Build history of the part. All positions in model axes, mm. A direction names the side the tool comes from. Round coordinates to 2 decimals unless told otherwise and drop trailing zeros. Write each loop counter-clockwise with the first axis right and the second up, starting at its lowest first coordinate (ties: lowest second). Pieces come first, ordered by that corner, then holes. Notation, with made-up numbers: M 26,60.25 L 65,60.25 A12 cw 65,69.25 Z; hole C 9,61.25 d4. An arc over 180 degrees is marked long. Write item = value, one per line.
from build123d import *

# Parameters (mm, degrees)
SKETCH_1_R      = 2.05
SKETCH_1_R_2    = 3
SKETCH_1_R_3    = 1.25
SKETCH_1_W      = 2.1
SKETCH_1_H      = 8.1
EXTRUDE_1_DEPTH = 2
FILLET_1_R      = 1.3
FILLET_2_R      = 2


with BuildPart() as part:
    # 草图1 → 凸台-拉伸1 (new body)
    with BuildSketch(Plane.XY):
        with BuildLine():
            Line((32.115707856, 28), (32.115707856, 22.85))
            Line((32.115707856, 22.85), (30.015707856, 22.85))
            Line((30.015707856, 22.85), (30.015707856, 28))
            Line((30.015707856, 28), (-29.075, 28))
            Line((-29.075, 28), (-38.998995168, 22.002009663))
            ThreePointArc((-38.998995168, 22.002009663), (-52.370174504, 17.472835843), (-60.236366221, 5.75))
            Line((-60.236366221, 5.75), (-79.631279411, 5.75))
            Line((-79.631279411, 5.75), (-79.631279411, -5.75))
            Line((-79.631279411, -5.75), (-60.236366221, -5.75))
            ThreePointArc((-60.236366221, -5.75), (-52.370174504, -17.472835843), (-38.998995168, -22.002009663))
            Line((-38.998995168, -22.002009663), (-29.075, -28))
            Line((-29.075, -28), (30.015707856, -28))
            Line((30.015707856, -28), (30.015707856, -22.85))
            Line((30.015707856, -22.85), (32.115707856, -22.85))
            Line((32.115707856, -22.85), (32.115707856, -28))
            Line((32.115707856, -28), (36.001004832, -28))
            Line((36.001004832, -28), (36.001004832, -26.017733681))
            Line((36.001004832, -26.017733681), (58.888331717, -26.017733681))
            Line((58.888331717, -26.017733681), (58.888331717, -21.401911511))
            Line((58.888331717, -21.401911511), (36.001004832, -21.401911511))
            Line((36.001004832, -21.401911511), (36.001004832, 28))
            Line((36.001004832, 28), (32.115707856, 28))
        make_face()
        with Locations((31.065707856, 15)):
            Circle(SKETCH_1_R, mode=Mode.SUBTRACT)
        with Locations(Location((31.065707856, -15, 0), (0, 0, 180))):
            Circle(SKETCH_1_R, mode=Mode.SUBTRACT)
        with Locations((-38.998995168, 0)):
            Circle(SKETCH_1_R_2, mode=Mode.SUBTRACT)
        with Locations((-38.998995168, -11.5)):
            Circle(SKETCH_1_R_3, mode=Mode.SUBTRACT)
        with Locations((-48.958287312, -5.75)):
            Circle(SKETCH_1_R_3, mode=Mode.SUBTRACT)
        with Locations((-48.958287312, 5.75)):
            Circle(SKETCH_1_R_3, mode=Mode.SUBTRACT)
        with Locations((-38.998995168, 11.5)):
            Circle(SKETCH_1_R_3, mode=Mode.SUBTRACT)
        with Locations((-29.039703025, 5.75)):
            Circle(SKETCH_1_R_3, mode=Mode.SUBTRACT)
        with Locations((-29.039703025, -5.75)):
            Circle(SKETCH_1_R_3, mode=Mode.SUBTRACT)
        with Locations((1.001004832, -25)):
            Circle(SKETCH_1_R, mode=Mode.SUBTRACT)
        with Locations((1.001004832, 25)):
            Circle(SKETCH_1_R, mode=Mode.SUBTRACT)
        with Locations((-74.958287312, 0)):
            Circle(SKETCH_1_R, mode=Mode.SUBTRACT)
        with Locations((31.065707856, 0)):
            Rectangle(SKETCH_1_W, SKETCH_1_H, mode=Mode.SUBTRACT)
        Polygon((2.100885183, -16.20323489), (23.065707856, -9.230000311), (23.065707856, 9.230000311), (2.100885183, 16.20323489), (-21.039703025, 1.3748119), (-21.039703025, -1.3748119), align=None, mode=Mode.SUBTRACT)
    extrude(amount=EXTRUDE_1_DEPTH)

    # 圆角1
    fillet_1_edges = [part.edges().sort_by_distance(p)[0] for p in [
        (-60.236366221, -5.75, 1),
        (-79.631279411, -5.75, 1),
        (-79.631279411, 5.75, 1),
        (-60.236366221, 5.75, 1),
        (30.015707856, 28, 1),
        (32.115707856, 28, 1),
        (32.115707856, -28, 1),
        (30.015707856, -28, 1),
    ]]
    fillet(fillet_1_edges, radius=FILLET_1_R)

    # 圆角2
    fillet_2_edges = [part.edges().sort_by_distance(p)[0] for p in [
        (-21.039703025, -1.3748119, 1),
        (2.100885183, -16.20323489, 1),
        (23.065707856, -9.230000311, 1),
        (23.065707856, 9.230000311, 1),
        (2.100885183, 16.20323489, 1),
        (-21.039703025, 1.3748119, 1),
    ]]
    fillet(fillet_2_edges, radius=FILLET_2_R)


solid = part.part
1. Band-saw the part on D-D (y = 25). List the corners of the cut face in (x, z), plus the area to 3 significant figures.
Responses:
outline = M -34.04,0 L -1.05,0 L -1.05,2 L -34.04,2 Z; M 3.05,0 L 30.02,0 L 30.02,2 L 3.05,2 Z; M 32.12,0 L 36,0 L 36,2 L 32.12,2 Z
area = 128 mm²
2. Flat gauge pins, fed straight in: pin 1 (1 mm diameter, centred on y = -6.5, z = 1.5, fed in from +X); pin 2 (0.6 mm diameter, centred on x = 46, z = 1, fed in from -Y); pin 3 (1 mm diameter, centred on x = 31, z = 1, fed in from -Y); pin 4 (2 mm diameter, centred on x = -29.04, y = 5.75, fed in from +Z). Where does each tip first touch, or does it go through?
Responses:
pin_1 = 36
pin_2 = -26.02
pin_3 = -22.85
pin_4 = through
3. Mould opens along Y. For faces 3 (the face through (-33.97, 25.04, 0.99)), 4 (the face through (-9.261, 8.923, 0.986)), 5 (the face through (-11, -12, 2)) say: pulls with the +Y half, pulls with the -Y half, needs draft (parallel to the pull), parting line crosses it, or undercut.
Responses:
face_3 = pulls with the +Y half
face_4 = undercut
face_5 = needs draft
4. Band-saw the part on A-A (x = -18). List the corners of the cut face in (y, z).
Responses:
outline = M -28,0 L -3.32,0 L -3.32,2 L -28,2 Z; M 3.32,0 L 28,0 L 28,2 L 3.32,2 Z
5. Band-saw the part on B-B (y = -11.5). List the corners of the cut face in (x, z).
Responses:
outline = M -57.76,0 L -40.25,0 L -40.25,2 L -57.76,2 Z; M -37.75,0 L -5.24,0 L -5.24,2 L -37.75,2 Z; M 16.24,0 L 36,0 L 36,2 L 16.24,2 Z
6. Band-saw the part on C-C (z = 0.45). Count the separate pieces of the cut face and the enclosed holes in it, plus the area to 3 significant figures.
Responses:
separate_pieces = 1
enclosed_holes = 14
area = 4,120 mm²
7. Tool access for faces 1 (the face through (-11, -12, 0)), 2 (the face through (12.48, 12.75, 0.99)): list every direction of +Z, -Z, +X, -X, +Y, -Y with a clear straight run to the whole face (end or side of a thin tool).
Responses:
face_1 = -Z, +X, -X, +Y, -Y
face_2 = +Z, -Z
8. Probe probe 1 along X at (y, z) = (-24, 1.5); probe 2 along Y at (x, z) = (16.5, 1.4); probe 3 along Y at (x, z) = (-4, 1.7). List the from-to ranges inside material, lowest first.
Responses:
probe_1 = -35.69 to -0.79, 2.79 to 30.02, 32.12 to 58.89
probe_2 = -28 to -11.41, 11.41 to 28
probe_3 = -28 to -12.29, 12.29 to 28
